```python
from build123d import *

# Parameters (mm, degrees)
MODEL_R         = 12
MODEL_R_2       = 2.625
EXTRUDE_1_DEPTH = 4


with BuildPart() as part:
    # Model → 凸台-拉伸1 (new body)
    with BuildSketch(Plane.XY):
        with BuildLine():
            Line((239.034732394, 334.032549296), (143.034732394, 334.032549296))
            ThreePointArc((143.034732394, 334.032549296), (141.620518832, 333.446762858), (141.034732394, 332.032549296))
            Line((141.034732394, 332.032549296), (141.034732394, 89.032549296))
            ThreePointArc((141.034732394, 89.032549296), (141.620518832, 87.618335733), (143.034732394, 87.032549296))
            Line((143.034732394, 87.032549296), (239.034732394, 87.032549296))
            ThreePointArc((239.034732394, 87.032549296), (240.448945957, 87.618335733), (241.034732394, 89.032549296))
            Line((241.034732394, 89.032549296), (241.034732394, 332.032549296))
            ThreePointArc((241.034732394, 332.032549296), (240.448945957, 333.446762858), (239.034732394, 334.032549296))
        make_face()
        with Locations((191.034732394, 157.032549296)):
            Circle(MODEL_R, mode=Mode.SUBTRACT)
        with Locations((177.034732394, 171.032549296)):
            Circle(MODEL_R_2, mode=Mode.SUBTRACT)
        with Locations((205.034732394, 171.032549296)):
            Circle(MODEL_R_2, mode=Mode.SUBTRACT)
        with Locations((177.034732394, 143.032549296)):
            Circle(MODEL_R_2, mode=Mode.SUBTRACT)
        with Locations((205.034732394, 143.032549296)):
            Circle(MODEL_R_2, mode=Mode.SUBTRACT)
        with Locations((149.034732394, 95.032549296)):
            Circle(MODEL_R_2, mode=Mode.SUBTRACT)
        with Locations((233.034732394, 95.032549296)):
            Circle(MODEL_R_2, mode=Mode.SUBTRACT)
        with Locations((149.034732394, 245.032549296)):
            Circle(MODEL_R_2, mode=Mode.SUBTRACT)
        with Locations((233.034732394, 245.032549296)):
            Circle(MODEL_R_2, mode=Mode.SUBTRACT)
        with Locations((149.034732394, 326.032549296)):
            Circle(MODEL_R_2, mode=Mode.SUBTRACT)
        with Locations((233.034732394, 326.032549296)):
            Circle(MODEL_R_2, mode=Mode.SUBTRACT)
        with Locations((191.034732394, 227.032549296)):
            Circle(MODEL_R_2, mode=Mode.SUBTRACT)
        with BuildLine():
            Line((217.159732394, 314.532549296), (217.159732394, 320.532549296))
            ThreePointArc((217.159732394, 320.532549296), (214.534732394, 323.157549296), (211.909732394, 320.532549296))
            Line((211.909732394, 320.532549296), (211.909732394, 314.532549296))
            ThreePointArc((211.909732394, 314.532549296), (214.534732394, 311.907549296), (217.159732394, 314.532549296))
        make_face(mode=Mode.SUBTRACT)
        with BuildLine():
            Line((217.159732394, 267.532549296), (217.159732394, 273.532549296))
            ThreePointArc((217.159732394, 273.532549296), (214.534732394, 276.157549296), (211.909732394, 273.532549296))
            Line((211.909732394, 273.532549296), (211.909732394, 267.532549296))
            ThreePointArc((211.909732394, 267.532549296), (214.534732394, 264.907549296), (217.159732394, 267.532549296))
        make_face(mode=Mode.SUBTRACT)
        with BuildLine():
            Line((172.034732394, 297.032549296), (172.034732394, 291.032549296))
            ThreePointArc((172.034732394, 291.032549296), (191.034732394, 272.032549296), (210.034732394, 291.032549296))
            Line((210.034732394, 291.032549296), (210.034732394, 297.032549296))
            ThreePointArc((210.034732394, 297.032549296), (191.034732394, 316.032549296), (172.034732394, 297.032549296))
        make_face(mode=Mode.SUBTRACT)
        with BuildLine():
            Line((170.159732394, 267.532549296), (170.159732394, 273.532549296))
            ThreePointArc((170.159732394, 273.532549296), (167.534732394, 276.157549296), (164.909732394, 273.532549296))
            Line((164.909732394, 273.532549296), (164.909732394, 267.532549296))
            ThreePointArc((164.909732394, 267.532549296), (167.534732394, 264.907549296), (170.159732394, 267.532549296))
        make_face(mode=Mode.SUBTRACT)
        with BuildLine():
            Line((170.159732394, 314.532549296), (170.159732394, 320.532549296))
            ThreePointArc((170.159732394, 320.532549296), (167.534732394, 323.157549296), (164.909732394, 320.532549296))
            Line((164.909732394, 320.532549296), (164.909732394, 314.532549296))
            ThreePointArc((164.909732394, 314.532549296), (167.534732394, 311.907549296), (170.159732394, 314.532549296))
        make_face(mode=Mode.SUBTRACT)
    extrude(amount=EXTRUDE_1_DEPTH)


solid = part.part
```
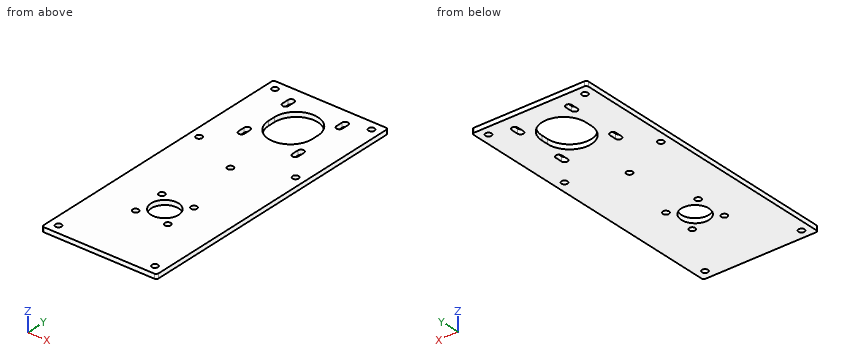
Verification items for the finished model (mm, model axes). Round coordinates to 2 decimals unless told otherwise and drop trailing zeros. Order: outer loops, then holes, each group sorted by start corner. A loop starts at its lowest first (then second) coordinate and runs counter-clockwise, first axis right, second up. Notation, with made-up numbers: (19.5, 75.5) - (33.5, 75.5) arc R23 ccw to (33.5, 92.5) - close; hole circle Ø9 at (-32.75, 59). An arc over 180 degrees is marked (long way). Use CSV: the item, a comma, the result in double quotes. Start each with the question number.
1) Section check A-A, the plane y = 305. Record the cut outline in (x, z), plus the area to 3 significant figures.
2) Section check D-D, the plane z = 1.65. State how many separate pieces and enclosed holes the cut face has, plus the area to 3 significant figures.
3) Section check C-C, the plane x = 186. Record the cut outline in (y, z).
4) Thickness scan on L1, parallel to Y at x = 149, z = 3.05; L2, parallel to Y at x = 192.5, z = 2.3; L3, parallel to Y at x = 213.5, z = 2.25 (3 decimals). Record the ranges inside material, lowest first.
5) Section check B-B, the plane x = 205.5. Record the cut outline in (y, z), plus the area to 3 significant figures.
Answers:
1,outline,"(141.03, 0) - (173.79, 0) - (173.79, 4) - (141.03, 4) - close; (208.28, 0) - (241.03, 0) - (241.03, 4) - (208.28, 4) - close"
1,area,"262 mm²"
2,separate pieces,"1"
2,enclosed holes,"17"
2,area,"22,400 mm²"
3,outline,"(87.03, 0) - (146.14, 0) - (146.14, 4) - (87.03, 4) - close; (167.93, 0) - (272.71, 0) - (272.71, 4) - (167.93, 4) - close; (315.35, 0) - (334.03, 0) - (334.03, 4) - (315.35, 4) - close"
4,L1,"y = 87.03 to 92.41, 97.66 to 242.41, 247.66 to 323.41, 328.66 to 334.03"
4,L2,"y = 87.03 to 145.12, 168.94 to 224.85, 229.21 to 272.09, 315.98 to 334.03"
4,L3,"y = 87.033 to 265.12, 275.945 to 312.12, 322.945 to 334.033"
5,outline,"(87.03, 0) - (140.45, 0) - (140.45, 4) - (87.03, 4) - close; (145.62, 0) - (168.45, 0) - (168.45, 4) - (145.62, 4) - close; (173.62, 0) - (278.71, 0) - (278.71, 4) - (173.62, 4) - close; (309.35, 0) - (334.03, 0) - (334.03, 4) - (309.35, 4) - close"
5,area,"824 mm²"
